Input: part model. Units: mm. Frame: model coordinates. A direction names the side the tool comes from. Give positions to 0.01 mm unless a question says otherwise; leave off trailing zeros. Loops run counter-clockwise (first coordinate to the right, second up) from the corner with the lowest first, then second, coordinate; pieces in that order, holes last. Notation, with made-up numbers: M 47.25,16 L 54.25,16 A30 ccw 54.25,40 Z; hole C 63.25,68 d10. An arc over 180 degrees is marked long. Answer as a JSON object with one key per item and string values. Group by question number.
1) First-contact query: P1, Ø1, axis at x = 132, y = 169, coming from the +Z side; P2, Ø9.5, axis at y = 198, z = 50.783, coming from the +X side; P3, Ø5, axis at y = 98, z = 50.783, coming from the -X side. Flat tips, straight axial feed; report the tip coordinate or a pass-through.
2) Ray query, L1, parallel to Z at x = 121, y = 32.1; L2, parallel to X at y = 164.5, z = -6.5; L3, parallel to X at y = 189, z = -160. Return the intervals inside material, ascending.
3) Draft query along Y for faces 3 (the flat face through (121, 0, -46)), 4 (the cylindrical face through (120.81, 95.619, 48.958)), 5 (the flat face through (140, 144, -162.217)). Return one class per face: +Y half, -Y half, draft (parallel to the pull), parting line (faces both ways), or undercut.
4) Section query B-B on z = -62. Return loops of the section in (x, y), plus the area to 3 significant figures.
5) Access query for faces 1 (the cylindrical face through (120.81, 199.38, 48.12)), 2 (the flat face through (122.289, 144, -44)). Directions: +Z, -Z, +X, -X, +Y, -Y. A direction counts if a zero-diameter tool reaches every point of the face in a straight line with its end or side. Return the directions, or none.
6) Section query A-A on y = 229. Return loops of the section in (x, z).
from build123d import *

# Parameters (mm, degrees)
F1_DEPTH = 293
F3_D     = 5
F5_D     = 6
F6_SIZE  = 2
F7_SIZE  = 2


with BuildPart() as f1:
    # F0 (on Front) → F1 (new body)
    with BuildSketch(Plane.XZ):
        with BuildLine():
            Line((122.288967, -156.216999), (122.288967, 70.783001))
            Line((122.288967, 70.783001), (119.288967, 70.783001))
            Line((119.288967, 70.783001), (119.288967, -156.216999))
            ThreePointArc((119.288967, -156.216999), (121.046326, -160.45964), (125.288967, -162.216999))
            Line((125.288967, -162.216999), (154.288967, -162.216999))
            Line((154.288967, -162.216999), (154.288967, -159.216999))
            Line((154.288967, -159.216999), (125.288967, -159.216999))
            ThreePointArc((125.288967, -159.216999), (123.167647, -158.338319), (122.288967, -156.216999))
        make_face()
    extrude(amount=-F1_DEPTH)

    # F3 (through all)
    with Locations(Plane.XY.offset(-159.216999)):
        with Locations((136.788967, 189), (136.788967, 211)):
            Hole(F3_D / 2)

    # F5 (through all)
    with Locations(Plane(origin=(119.288967, 0, 0), x_dir=(0, -1, 0), z_dir=(-1, 0, 0))):
        with Locations((-32.1, 55.783001), (-32.1, -114.216999), (-263.9, -114.216999), (-263.9, 55.783001), (-98, 50.783001), (-198, 50.783001)):
            Hole(F5_D / 2)

    # F6
    f6_edges = [f1.edges().sort_by_distance(p)[0] for p in [
        (120.788967, 0, 70.783001),
        (120.788967, 293, 70.783001),
        (154.288967, 293, -160.716999),
    ]]
    chamfer(f6_edges, length=F6_SIZE)

    # F7
    f7_edges = [f1.edges().sort_by_distance(p)[0] for p in [
        (154.288967, 0, -160.716999),
    ]]
    chamfer(f7_edges, length=F7_SIZE)


solid = f1.part
Output:
{
 "1": {"P1": "stops at z = -159.22", "P2": "stops at x = 122.29", "P3": "passes through"},
 "2": {"L1": "z = -160.41 to -117.22, -111.22 to 52.78, 58.78 to 70.78", "L2": "x = 119.29 to 122.29", "L3": "x = 120.63 to 134.29, 139.29 to 154.29"},
 "3": {"face 3": "-Y half", "face 4": "undercut", "face 5": "draft"},
 "4": {"outline": "M 119.29,0 L 122.29,0 L 122.29,293 L 119.29,293 Z", "area": "879 mm^2"},
 "5": {"face 1": "+X, -X", "face 2": "+Z, +X, +Y, -Y"},
 "6": {"outline": "M 119.29,-156.22 A6 ccw 125.29,-162.22 L 154.29,-162.22 L 154.29,-159.22 L 125.29,-159.22 A3 cw 122.29,-156.22 L 122.29,70.78 L 119.29,70.78 Z"}
}
